```python
from build123d import *

# Parameters (mm, degrees)
BOSS_EXTRUDE1_DEPTH         = 100
TAP_DRILL_FOR_M6X1_0_TAP1_D = 5


with BuildPart() as part:
    # Sketch1 → Boss-Extrude1 (new body)
    with BuildSketch(Plane(origin=(0, 0, 0), x_dir=(0, 0, -1), z_dir=(1, 0, 0))):
        Polygon((0, 25), (0, 0), (8, 0), (8, 20), (5, 20), (5, 25), align=None)
    extrude(amount=BOSS_EXTRUDE1_DEPTH)

    # Tap Drill for M6x1.0 Tap1 (through all)
    with Locations(Plane(origin=(87, 12.5, 0), x_dir=(1, 0, 0), z_dir=(0, 0, 1))):
        with Locations((0, 0), (-74, 0)):
            Hole(TAP_DRILL_FOR_M6X1_0_TAP1_D / 2)


solid = part.part
```
Geometry check sheet. Reference: the model listing, model coordinates, mm. A direction names the side the tool comes from. Round coordinates to 2 decimals unless told otherwise and drop trailing zeros. Order: outer loops, then holes, each group sorted by start corner. A loop starts at its lowest first (then second) coordinate and runs counter-clockwise, first axis right, second up. Notation, with made-up numbers: (42, -1.5) -> (96, -1.5) arc R14 cw to (96, 5.5) -> close; hole circle Ø9 at (-4.75, 36.5). An arc over 180 degrees is marked (long way). Return JSON: item names as keys, results as strings. Group by question number.
Q1. Section check B-B, the plane z = -6.5. Record the boundary of the cut face in (x, y).
Q2. Section check C-C, the plane y = 11.5. Record the boundary of the cut face in (x, z).
Q3. Section check D-D, the plane x = 86. Record the boundary of the cut face in (y, z), plus the area to 3 significant figures.
Q4. Gauge pin test, flat end, axial feed: pin 1 (4 mm diameter, centred on x = 27, y = 23.5, fed in from -Z). Record the tip position at first contact, or that the pin passes through.
Q5. Tool access check on faces 4 (the flat face through (49, 13, 0)), 5 (the flat face through (49, 22, -5)). Record the directions out of +Z, -Z, +X, -X, +Y, -Y that give a thin tool (end or side, any length) a straight path to the whole face; none if there is none.
Q6. Material ranges on probe 1 along Y at (x, z) = (13, -3.75); probe 2 along Y at (x, z) = (87, -5.25); probe 3 along Y at (x, z) = (95.5, -5.5), recorded low to high. Write a range as from..to.
Q7. Section check A-A, the plane x = 13. Record the boundary of the cut face in (y, z), plus the area to 3 significant figures.
Q8. Release check for a two-part mould opening along Y. For faces 1 (the flat face through (49, 0, -4)), 2 (the flat face through (49, 25, -3)), 3 (the cylindrical face through (13.54, 10.06, -4.06)) record: released by +Y, released by -Y, zero draft, split by the parting line, or undercut.
Numbers:
{
 "1": {"outline": "(0, 0) -> (100, 0) -> (100, 20) -> (0, 20) -> close; hole circle Ø5 at (13, 12.5); hole circle Ø5 at (87, 12.5)"},
 "2": {"outline": "(0, -8) -> (10.71, -8) -> (10.71, 0) -> (0, 0) -> close; (15.29, -8) -> (84.71, -8) -> (84.71, 0) -> (15.29, 0) -> close; (89.29, -8) -> (100, -8) -> (100, 0) -> (89.29, 0) -> close"},
 "3": {"outline": "(0, -8) -> (10.21, -8) -> (10.21, 0) -> (0, 0) -> close; (14.79, -8) -> (20, -8) -> (20, -5) -> (25, -5) -> (25, 0) -> (14.79, 0) -> close", "area": "148 mm^2"},
 "4": {"pin 1": "z = -5"},
 "5": {"face 4": "+Z, +X, -X, +Y, -Y", "face 5": "-Z, +X, -X, +Y"},
 "6": {"probe 1": "0..10, 15..25", "probe 2": "0..10, 15..20", "probe 3": "0..20"},
 "7": {"outline": "(0, -8) -> (10, -8) -> (10, 0) -> (0, 0) -> close; (15, -8) -> (20, -8) -> (20, -5) -> (25, -5) -> (25, 0) -> (15, 0) -> close", "area": "145 mm^2"},
 "8": {"face 1": "released by -Y", "face 2": "released by +Y", "face 3": "undercut"}
}
